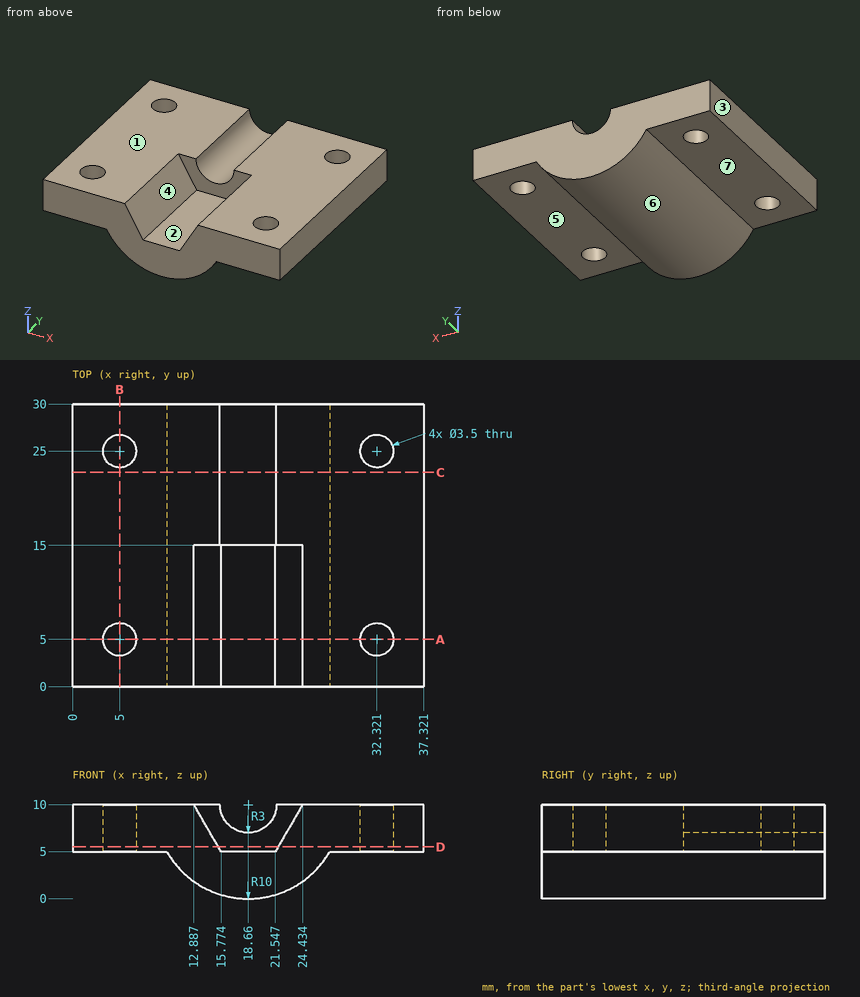
Verification items for this drawing (mm, ordinates from the low corner). A direction names the side the tool comes from. Give positions to 0.01 mm unless a question says otherwise; leave off trailing zeros. Loops run counter-clockwise (first coordinate to the right, second up) from the corner with the lowest first, then second, coordinate; pieces in that order, holes last. Notation, with made-up numbers: M 83,49.5 L 105,49.5 A18 ccw 105,69.5 Z; hole C -14.75,15.5 d4. An arc over 180 degrees is marked long. Answer as a JSON object with one key per item and string values. Group by question number.
Item 1: Sectioned sample at A-A on y = 5. Record the boundary of the cut face in (x, z).
Item 2: Gauge pin test, flat ends, axial feed: pin 1 (5 mm diameter, centred on x = 6.5, y = 14, fed in from -Z); pin 2 (1.7 mm diameter, centred on x = 19.5, y = 9, fed in from +Z). Record the tip position at first contact, or that the pin passes through.
Item 3: Sectioned sample at D-D on z = 5.5. Give the number of separate pieces and of enclosed holes in the cut face, plus the area to 3 significant figures.
Item 4: Access from +Z, -Z, +X, -X, +Y, -Y to the whole of each face (thin tool, end or side, straight path). Record for the marked faces 4, 5, 6 and 7.
Item 5: Sectioned sample at C-C on y = 22.75. Record the boundary of the cut face in (x, z), plus the area to 3 significant figures.
Item 6: Mould release check, pull along X, two halves, no side actions. Record for the marked faces 1, 2 and 3: pulls with the +X half, pulls with the -X half, needs draft (parallel to the pull), parting line crosses it, or undercut.
Item 7: Material ranges on L1, parallel to Y at x = 5, z = 7.35; L2, parallel to X at y = 25.25, z = 9; L3, parallel to Z at x = 30.5, y = 25.75, recorded low to high.
Item 8: Sectioned sample at B-B on x = 5. Record the boundary of the cut face in (y, z).
Findings below:
{
 "1": {"outline": "M 0,5 L 3.25,5 L 3.25,10 L 0,10 Z; M 6.75,5 L 10,5 A10 ccw 27.32,5 L 30.57,5 L 30.57,10 L 24.43,10 L 21.55,5 L 15.77,5 L 12.89,10 L 6.75,10 Z; M 34.07,5 L 37.32,5 L 37.32,10 L 34.07,10 Z"},
 "2": {"pin 1": "z = 5", "pin 2": "z = 5"},
 "3": {"separate pieces": "1", "enclosed holes": "4", "area": "986 mm2"},
 "4": {"face 4": "+Z, -Y", "face 5": "-Z, +X, +Y, -Y", "face 6": "-Z, +Y, -Y", "face 7": "-Z, -X, +Y, -Y"},
 "5": {"outline": "M 0,5 L 10,5 A10 ccw 27.32,5 L 37.32,5 L 37.32,10 L 21.66,10 A3 cw 15.66,10 L 0,10 Z", "area": "234 mm2"},
 "6": {"face 1": "needs draft", "face 2": "undercut", "face 3": "pulls with the -X half"},
 "7": {"L1": "0 to 3.25, 6.75 to 23.25, 26.75 to 30", "L2": "0 to 3.27, 6.73 to 15.83, 21.49 to 30.59, 34.05 to 37.32", "L3": "5 to 10"},
 "8": {"outline": "M 0,5 L 3.25,5 L 3.25,10 L 0,10 Z; M 6.75,5 L 23.25,5 L 23.25,10 L 6.75,10 Z; M 26.75,5 L 30,5 L 30,10 L 26.75,10 Z"}
}
